Can you work these out from the model? Positions are in its coordinate system, mm. A direction names the side the tool comes from. Give positions to 0.01 mm unless a question says otherwise; leave off trailing zeros. Order: outer loops, then holes, each group sorted by start corner. A loop starts at its lowest first (then second) coordinate and runs counter-clockwise, first axis right, second up. Notation, with made-up numbers: (-11, 54) - (-7, 54) arc R15 cw to (-7, 71) - close; hole circle Ø9 at (8.25, 72). An arc over 180 degrees is marked (long way). Answer as a JSON object with one key per item and string values.
```python
from build123d import *

# Parameters (mm, degrees)
F0_R        = 25
F1_DEPTH    = 65.5
F2_R        = 8
F3_DEPTH    = 44
F4_W        = 17.7049817399
F4_H        = 63.7933180105
F4_W_2      = 20.9798936745
F4_H_2      = 49.4306737048
F5_DEPTH    = 49.3
F6_C1_SIZE2 = 2.3094010768
F6_C1_SIZE  = 4
F6_C2_SIZE2 = 4
F6_C2_SIZE  = 2.3094010768
F7_R        = 27.6347360806
F7_R_2      = 12.45
F8_DEPTH    = 25.5
F9_R        = 2
F11_DEPTH   = 44.3
F12_C1_SIZE = 7
F12_C2_SIZE = 6.9999
F13_R       = 10.1
F14_DEPTH   = 4.5
F15_R       = 10.1
F16_DEPTH   = 4.5
F17_R       = 7.5
F18_DEPTH   = 16.5
F19_R       = 7.5
F20_DEPTH   = 16.5


# Not quite as in the source:
# - a fillet or chamfer is up to 0.001 mm smaller than in the source, because OpenCascade refuses the exact size


with BuildPart() as f1:
    # F0 (on Top) → F1 (new body)
    with BuildSketch(Plane.XY):
        Circle(F0_R)
    extrude(amount=F1_DEPTH)

    # F2 (on face) → F3 (cut)
    with BuildSketch(Plane(origin=(0, 0, 0), x_dir=(1, 0, 0), z_dir=(0, 0, -1))):
        Circle(F2_R)
    extrude(amount=-F3_DEPTH, mode=Mode.SUBTRACT)

    # F4 (on Front) → F5 (cut, symmetric)
    with BuildSketch(Plane.XZ):
        with Locations((28.8524908699, 55.8966590053)):
            Rectangle(F4_W, F4_H)
        with Locations((-30.4899468372, 48.7153368524)):
            Rectangle(F4_W_2, F4_H_2)
    extrude(amount=F5_DEPTH, both=True, mode=Mode.SUBTRACT)

    # F6: chamfer of 4 x 2.3094010768 on 2 edges, made by hand

    # F6_c1
    f6_c1_edges = [f1.edges().sort_by_distance(p)[0] for p in [
        (20, 0, 65.5),
    ]]
    f6_c1_side = f1.faces().sort_by_distance((20, 0, 65.4538119785))[0]
    chamfer(f6_c1_edges, length=F6_C1_SIZE, length2=F6_C1_SIZE2, reference=f6_c1_side)

    # F6_c2
    f6_c2_edges = [f1.edges().sort_by_distance(p)[0] for p in [
        (-20, 0, 65.5),
    ]]
    f6_c2_side = f1.faces().sort_by_distance((-19.9538119785, 0, 65.5))[0]
    chamfer(f6_c2_edges, length=F6_C2_SIZE, length2=F6_C2_SIZE2, reference=f6_c2_side)

    # F7 (on face) → F8 (cut)
    with BuildSketch(Plane(origin=(0, 0, 0), x_dir=(1, 0, 0), z_dir=(0, 0, -1))):
        Circle(F7_R)
        Circle(F7_R_2, mode=Mode.SUBTRACT)
    extrude(amount=-F8_DEPTH, mode=Mode.SUBTRACT)

    # F9
    f9_edges = [f1.edges().sort_by_distance(p)[0] for p in [
        (-12.45, 0, 25.5),
    ]]
    fillet(f9_edges, radius=F9_R)

    # F10 (on Right) → F11 (cut, symmetric)
    with BuildSketch(Plane.YZ):
        Polygon((2.7942564781, 69.2223283856), (14.0074999573, 53.2081570616), (27.8284827581, 33.4697480234), (27.8284827581, 71.2105557323), align=None)
        Polygon((-28.691531344, 32.2371869058), (-14.0074999573, 53.2081570616), (-2.0273737507, 70.3175504242), (-27.1908640862, 71.7121362686), align=None)
    extrude(amount=F11_DEPTH, both=True, mode=Mode.SUBTRACT)

    # F12: chamfer of 7 on 3 edges, made by hand

    # F12_c1
    f12_c1_edges = [f1.edges().sort_by_distance(p)[0] for p in [
        (0, 25, 25.5),
    ]]
    chamfer(f12_c1_edges, length=F12_C1_SIZE)

    # F12_c2 (size 7 in the source; OpenCascade refuses exactly that, so slightly less here)
    f12_c2_edges = [f1.edges().sort_by_distance(p)[0] for p in [
        (0, -25, 25.5),
    ]]
    chamfer(f12_c2_edges, length=F12_C2_SIZE)

    # F13 (on face) → F14 (cut)
    with BuildSketch(Plane(origin=(0, -34.3988298284, 24.0863199514), x_dir=(1, 0, 0), z_dir=(0, -0.8191520443, 0.5735764364))):
        with Locations((0, 35.2567682304)):
            Circle(F13_R)
    extrude(amount=-F14_DEPTH, mode=Mode.SUBTRACT)

    # F15 (on face) → F16 (cut)
    with BuildSketch(Plane(origin=(0, 34.3988298284, 24.0863199514), x_dir=(-1, 0, 0), z_dir=(0, 0.8191520443, 0.5735764364))):
        with Locations((0, 35.2567682304)):
            Circle(F15_R)
    extrude(amount=-F16_DEPTH, mode=Mode.SUBTRACT)

    # F17 (on face) → F18 (cut)
    with BuildSketch(Plane(origin=(0, 30.7126456291, 21.5052259879), x_dir=(-1, 0, 0), z_dir=(0, 0.8191520443, 0.5735764364))):
        with Locations((0, 35.2567682304)):
            Circle(F17_R)
    extrude(amount=-F18_DEPTH, mode=Mode.SUBTRACT)

    # F19 (on face) → F20 (cut)
    with BuildSketch(Plane(origin=(0, -30.7126456291, 21.5052259879), x_dir=(1, 0, 0), z_dir=(0, -0.8191520443, 0.5735764364))):
        with Locations((0, 35.2567682304)):
            Circle(F19_R)
    extrude(amount=-F20_DEPTH, mode=Mode.SUBTRACT)


solid = f1.part
```
Q1. If we section it at A-A, the plane x = 0: Count the separate pieces of the cut face and the enclosed holes in it, then the cut area to 3 significant figures.
Recorded:
{"separate pieces": "3", "enclosed holes": "0", "area": "886 mm^2"}
Q2. If we section it at D-D, the plane z = 15: Please give me the cut outline in (x, y).
Recorded:
{"outline": "circle Ø24.9 at (0, 0); hole circle Ø16 at (0, 0)"}
Q3. Which directions (+Z, -Z, +X, -X, +Y, -Y) give clear straight access to the entire face, cutting with the end or side of a thin tool? Please do faces 1 (the face through (-9.18, -8.41, 11.59)), 2 (the face through (-1.543, -6.172, 56.553)), 3 (the face through (-0.3, 20, 27.5)).
Recorded:
{"face 1": "-Z", "face 2": "none", "face 3": "-Z, +Y"}
Q4. I need wall thicknesses on L1, parallel to X at y = 0, z = 34; L2, parallel to X at y = 0, z = 23. Which ranges of each line are inside material? Lowest first, please.
Recorded:
{"L1": "x = -20 to -8, 8 to 20", "L2": "x = -12.45 to -8, 8 to 12.45"}
Q5. I'm going to push flat-ended pins straight in: pin 1 Ø1.5 at (x, y) = (4.5, -14.5) entering from -Z; pin 2 Ø0.6 at (x, y) = (-7.5, -1) entering from -Z; pin 3 Ø12 at (y, z) = (-10, 18.5) entering from +X. Where does each tip first touch, or does it pass through?
Recorded:
{"pin 1": "stops at z = 25.5", "pin 2": "stops at z = 44", "pin 3": "stops at x = 11.79"}
Q6. We'd pull the mould along Y, two halves only. Please class faces 4 (the face through (-18.861, -0.115, 63.472)), 5 (the face through (0, 25, 36)), 6 (the face through (-2.189, -18.014, 43.618)): released by +Y, released by -Y, zero draft, split by the parting line, or undercut.
Recorded:
{"face 4": "zero draft", "face 5": "released by +Y", "face 6": "undercut"}
Q7. If we section it at B-B, the plane z = 36: Please give me the cut outline in (x, y).
Recorded:
{"outline": "(-20, -15) arc R25 ccw to (20, -15) - (20, 15) arc R25 ccw to (-20, 15) - close; hole circle Ø16 at (0, 0)"}
